CAD build for the part. Positions are in the model's coordinates, mm. Round coordinates to 2 decimals unless told otherwise and drop trailing zeros. Loops run counter-clockwise (first coordinate to the right, second up) from the corner with the lowest first, then second, coordinate; pieces in that order, holes last. Notation, with made-up numbers: M 30,8.25 L 85,8.25 A19 ccw 85,17.25 Z; hole C -13,-7.5 d10. An arc over 180 degrees is marked long. Use one line per item in the form item = value.
from build123d import *

# Parameters (mm, degrees)
SKETCH_1_R          = 3.25
SKETCH_1_R_2        = 7.5
EXTRUDE_1_DEPTH     = 4
SKETCH_2_W          = 1
SKETCH_2_H          = 19.943647813
CUT_EXTRUDE_1_DEPTH = 46
CHAMFER_1_SIZE      = 3
CHAMFER_2_SIZE      = 0.5


with BuildPart() as part:
    # Эскиз1 → Бобышка-Вытянуть1 (new body)
    with BuildSketch(Plane.XY):
        with BuildLine():
            Line((20, 69.629043508), (20, 400))
            Line((20, 400), (-20, 400))
            Line((-20, 400), (-20, 69.629043508))
            ThreePointArc((-20, 69.629043508), (-15.501661364, 54.765331367), (-20.05985163, 39.919864362))
            ThreePointArc((-20.05985163, 39.919864362), (0, 0), (20.05985163, 39.919864362))
            ThreePointArc((20.05985163, 39.919864362), (15.501661364, 54.765331367), (20, 69.629043508))
        make_face()
        with Locations((0, 370)):
            Circle(SKETCH_1_R, mode=Mode.SUBTRACT)
        with Locations((0, 350)):
            Circle(SKETCH_1_R, mode=Mode.SUBTRACT)
        with Locations((0, 25)):
            Circle(SKETCH_1_R_2, mode=Mode.SUBTRACT)
    extrude(amount=EXTRUDE_1_DEPTH)

    # Эскиз2 → Вырез-Вытянуть1 (cut, through all)
    with BuildSketch(Plane.ZY.offset(20)):
        with Locations((3.5, 390.028176094)):
            Rectangle(SKETCH_2_W, SKETCH_2_H)
    extrude(amount=-CUT_EXTRUDE_1_DEPTH, mode=Mode.SUBTRACT)

    # Фаска1
    chamfer_1_edges = [part.edges().sort_by_distance(p)[0] for p in [
        (-3.25, 370, 0),
    ]]
    chamfer(chamfer_1_edges, length=CHAMFER_1_SIZE)

    # Фаска2
    chamfer_2_edges = [part.edges().sort_by_distance(p)[0] for p in [
        (-3.25, 350, 0),
        (-3.25, 350, 4),
        (-3.25, 370, 4),
    ]]
    chamfer(chamfer_2_edges, length=CHAMFER_2_SIZE)


solid = part.part
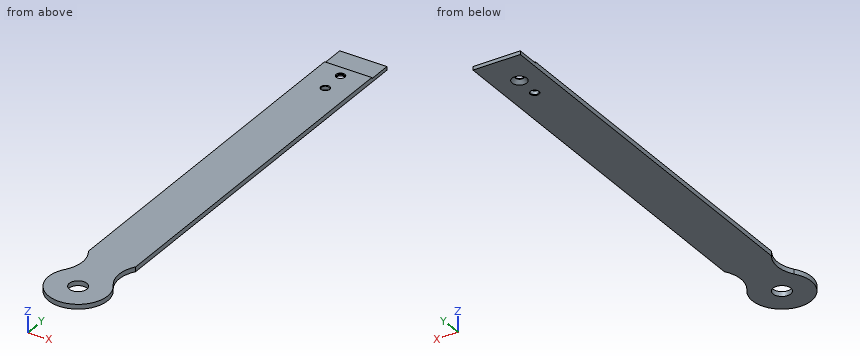
1. Drop flat-ended pins along their axis: P1, Ø0.5, axis at x = -9, z = 3.5, coming from the +Y side; P2, Ø10.5, axis at x = 0, y = 350, coming from the -Z side; P3, Ø10, axis at x = 5, y = 385.5, coming from the +Z side; P4, Ø13.5, axis at x = 0, y = 25, coming from the -Z side (3 decimals). Give the stop position or say it passes through.
Completed:
P1 = 380.06
P2 = 0
P3 = 3
P4 = through
2. Cut at D-D on y = 25. Write the cut outline in (x, z).
Completed:
outline = M -25,0 L -7.5,0 L -7.5,4 L -25,4 Z; M 7.5,0 L 25,0 L 25,4 L 7.5,4 Z
3. Cut at A-A on z = 2.2. Write the cut outline in (x, y).
Completed:
outline = M -20.06,39.92 A25 ccw long 20.06,39.92 A26.63 cw 20,69.63 L 20,400 L -20,400 L -20,69.63 A26.63 cw Z; hole C 0,25 d15; hole C 0,370 d8.1; hole C 0,350 d6.5
4. Probe line 1 along Y through (x, z) = (0, 3.2); line 2 along X through (y, z) = (370, 3.35); line 3 along Y through (x, z) = (0, 1.8). List the from-to ranges inside material, lowest first. Write a range as from..to.
Completed:
line_1 = 0..17.5, 32.5..346.75, 353.25..366.75, 373.25..380.06
line_2 = -20..-3.25, 3.25..20
line_3 = 0..17.5, 32.5..346.75, 353.25..365.55, 374.45..400
5. Cut at B-B on y = 350. Write the cut outline in (x, z).
Completed:
outline = M -20,0 L -3.75,0 L -3.25,0.5 L -3.25,3.5 L -3.75,4 L -20,4 Z; M 3.25,0.5 L 3.75,0 L 20,0 L 20,4 L 3.75,4 L 3.25,3.5 Z
6. Cut at C-C on x = 0. Write the cut outline in (y, z), and give its area (3 significant figures).
Completed:
outline = M 0,0 L 17.5,0 L 17.5,4 L 0,4 Z; M 32.5,0 L 346.25,0 L 346.75,0.5 L 346.75,3.5 L 346.25,4 L 32.5,4 Z; M 353.25,0.5 L 353.75,0 L 363.75,0 L 366.75,3 L 366.75,3.5 L 366.25,4 L 353.75,4 L 353.25,3.5 Z; M 373.25,3 L 376.25,0 L 400,0 L 400,3 L 380.06,3 L 380.06,4 L 373.75,4 L 373.25,3.5 Z
area = 1,460 mm2
